Geometry: final body of the model. Coordinates: model frame, mm. A direction names the side the tool comes from. Give positions to 0.01 mm unless a question says otherwise; leave off trailing zeros. Write each loop counter-clockwise with the first axis right and the second up, starting at its lowest first coordinate (ties: lowest second). Pieces come first, ordered by that corner, then holes. Notation, with made-up numbers: (85.5, 32.25) -> (115.5, 32.25) arc R14 cw to (115.5, 37.25) -> close; hole circle Ø1 at (21.25, 83). An arc over 180 degrees is marked (long way). Answer as a JSON object with one key per item and string values.
from build123d import *

# Parameters (mm, degrees)
F0_W     = 96.46225
F0_H     = 5.296454
F0_W_2   = 88.428333
F0_H_2   = 155.114882
F1_DEPTH = 25.4
F2_R     = 23.151618
F3_DEPTH = 65.394416
F4_R     = 6.73018
F5_DEPTH = 25.4


with BuildPart() as f1:
    # F0 (on Front) → F1 (new body)
    with BuildSketch(Plane.XZ):
        with Locations((-48.231125, 98.453775)):
            Rectangle(F0_W, F0_H)
        with Locations((44.214166, 98.453775)):
            Rectangle(F0_W_2, F0_H)
        with Locations((44.214166, 18.248107)):
            Rectangle(F0_W_2, F0_H_2)
    extrude(amount=F1_DEPTH)

    # F2 (on Front) → F3 (join)
    with BuildSketch(Plane.XZ):
        with Locations((44.85137, 20.544406)):
            Circle(F2_R)
    extrude(amount=F3_DEPTH)

    # F4 (on face) → F5 (join)
    with BuildSketch(Plane.XZ.offset(65.394416)):
        with Locations((48.735432, 25.047414)):
            Circle(F4_R)
    extrude(amount=F5_DEPTH)


solid = f1.part
Q1. Cut plane D-D (z = 0). Return the cut outline in (x, y), and give its area (3 significant figures).
Values:
{"outline": "(0, -25.4) -> (34.18, -25.4) -> (34.18, -65.39) -> (55.52, -65.39) -> (55.52, -25.4) -> (88.43, -25.4) -> (88.43, 0) -> (0, 0) -> close", "area": "3,100 mm²"}
Q2. Cut plane C-C (x = -80). Return the cut outline in (y, z).
Values:
{"outline": "(-25.4, 95.81) -> (0, 95.81) -> (0, 101.1) -> (-25.4, 101.1) -> close"}
Q3. Material intervals for L1, parallel to Y at x = 56, z = -21.5; L2, parallel to Z at x = -42.5, y = -5.5; L3, parallel to X at y = -11.5, z = 44, sorted ascending. Write a range as from..to.
Values:
{"L1": "-25.4..0", "L2": "95.81..101.1", "L3": "0..88.43"}
Q4. Cut plane B-B (z = 84.5). Return the cut outline in (x, y), and give its area (3 significant figures).
Values:
{"outline": "(0, -25.4) -> (88.43, -25.4) -> (88.43, 0) -> (0, 0) -> close", "area": "2,250 mm²"}
Q5. First-contact query: P1, Ø12.5, axis at x = -26, y = -13.5, coming from the -Z side; P2, Ø12.5, axis at y = -16, z = -0.5, coming from the -X side; P3, Ø2, axis at x = 67, z = -11, coming from the -Y side. Flat tips, straight axial feed; report the tip coordinate or a pass-through.
Values:
{"P1": "z = 95.81", "P2": "x = 0", "P3": "y = -25.4"}
Q6. Set-up query: faces 1 (the flat face through (49, -90.794, 25)), 2 (the flat face through (0, -13, 17)), 3 (the cylindrical face through (42.01, -77.92, 25.34)). Return all of +Z, -Z, +X, -X, +Y, -Y with unobstructed straight access to the full face (end or side cutting, diameter ignored); none if empty.
Values:
{"face 1": "+Z, -Z, +X, -X, -Y", "face 2": "-Z, -X, +Y, -Y", "face 3": "-Y"}
Q7. Cut plane A-A (y = -23). Return the cut outline in (x, z), and give its area (3 significant figures).
Values:
{"outline": "(-96.46, 95.81) -> (0, 95.81) -> (0, -59.31) -> (88.43, -59.31) -> (88.43, 101.1) -> (-96.46, 101.1) -> close", "area": "14,700 mm²"}
